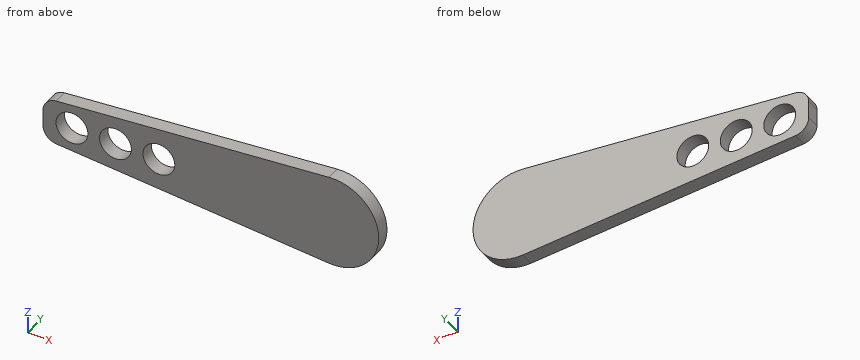
```python
from build123d import *

# Parameters (mm, degrees)
SKETCH2_R           = 5.5
SKETCH2_R_2         = 15.875
BOSS_EXTRUDE1_DEPTH = 4.7625
FILLET1_R           = 5


with BuildPart() as part:
    # Sketch2 → Boss-Extrude1 (new body)
    # profile 1 of 2: a face of its own
    with BuildSketch(Plane(origin=(0, 0, 0), x_dir=(1, 0, 0), z_dir=(0, 1, 0))):
        with BuildLine():
            ThreePointArc((-1.333740348, -15.818873591), (-15.875, -1.13e-07), (-1.333740574, 15.818873572))
            Line((-1.333740574, 15.818873572), (-100, 7.5))
            Line((-100, 7.5), (-100, -7.5))
            Line((-100, -7.5), (-1.333740348, -15.818873591))
        make_face()
        with Locations(Location((-90, 0, 0), (0, 0, 90))):
            Circle(SKETCH2_R, mode=Mode.SUBTRACT)
        with Locations(Location((-75, 0, 0), (0, 0, 90))):
            Circle(SKETCH2_R, mode=Mode.SUBTRACT)
        with Locations(Location((-60, 0, 0), (0, 0, 90))):
            Circle(SKETCH2_R, mode=Mode.SUBTRACT)
    # profile 2 of 2: a face of its own
    with BuildSketch(Plane(origin=(0, 0, 0), x_dir=(1, 0, 0), z_dir=(0, 1, 0))):
        Circle(SKETCH2_R_2)
    extrude(amount=BOSS_EXTRUDE1_DEPTH)

    # Fillet1
    fillet1_edges = [part.edges().sort_by_distance(p)[0] for p in [
        (-100, 2.38125, 7.5),
        (-100, 2.38125, -7.5),
    ]]
    fillet(fillet1_edges, radius=FILLET1_R)


solid = part.part
```
Here's how the part is built. I have some questions about the finished solid (model axes, mm). Coordinates: 2 decimals unless noted, no trailing zeros. Loops run counter-clockwise (first coordinate to the right, second up) from the corner with the lowest first, then second, coordinate; pieces in that order, holes last. Notation, with made-up numbers: (43.25, 76) - (47.25, 76) arc R14 ccw to (47.25, 97) - close; hole circle Ø1 at (50, 19). An arc over 180 degrees is marked (long way). Return JSON: item names as keys, results as strings. Group by question number.
Item 1: If we section it at A-A on z = 0: Write out the boundary of the cut face in (x, y) (1 decimal).
Item 2: If we section it at B-B on y = 1.2: Write out the boundary of the cut face in (x, z) (3 decimals).
Item 3: If we section it at C-C on x = -90: Write out the boundary of the cut face in (y, z).
Item 4: Will these pins go through, and if not, where does the flat tip stop? P1, Ø2, axis at y = 3.5, z = 9, coming from the +X side; P2, Ø1, axis at y = 2.5, z = -6, coming from the -X side.
Item 5: If we section it at D-D on z = 4.5: Write out the boundary of the cut face in (x, y), and give its area (3 significant figures).
Item 6: I need wall thicknesses on line 1 (X direction, y = 1.3, z = 0) (3 decimals); line 2 (X direction, y = 4.45, z = 5); line 3 (Z direction, x = -60, y = 2.5). Which ranges of each line are inside material? Lowest first, please. Write a range as from..to.
Calculated:
{
 "1": {"outline": "(-100, 0) - (-95.5, 0) - (-95.5, 4.8) - (-100, 4.8) - close; (-84.5, 0) - (-80.5, 0) - (-80.5, 4.8) - (-84.5, 4.8) - close; (-69.5, 0) - (-65.5, 0) - (-65.5, 4.8) - (-69.5, 4.8) - close; (-54.5, 0) - (15.9, 0) - (15.9, 4.8) - (-54.5, 4.8) - close"},
 "2": {"outline": "(-100, -2.904) arc R5 ccw to (-95.42, -7.886) - (-1.334, -15.819) arc R15.875 ccw (long way) to (-1.334, 15.819) - (-95.42, 7.886) arc R5 ccw to (-100, 2.904) - close; hole circle Ø11 at (-90, 0); hole circle Ø11 at (-75, 0); hole circle Ø11 at (-60, 0)"},
 "3": {"outline": "(0, -8.34) - (4.76, -8.34) - (4.76, -5.5) - (0, -5.5) - close; (0, 5.5) - (4.76, 5.5) - (4.76, 8.34) - (0, 8.34) - close"},
 "4": {"P1": "stops at x = 13.71", "P2": "stops at x = -99.27"},
 "5": {"outline": "(-99.74, 0) - (-93.16, 0) - (-93.16, 4.76) - (-99.74, 4.76) - close; (-86.84, 0) - (-78.16, 0) - (-78.16, 4.76) - (-86.84, 4.76) - close; (-71.84, 0) - (-63.16, 0) - (-63.16, 4.76) - (-71.84, 4.76) - close; (-56.84, 0) - (15.22, 0) - (15.22, 4.76) - (-56.84, 4.76) - close", "area": "457 mm^2"},
 "6": {"line 1": "x = -100..-95.5, -84.5..-80.5, -69.5..-65.5, -54.5..15.875", "line 2": "x = -99.54..-92.29, -87.71..-77.29, -72.71..-62.29, -57.71..15.07", "line 3": "z = -10.87..-5.5, 5.5..10.87"}
}
